For this review, take the finished solid that the model builds, in its own axes (mm). A direction names the side the tool comes from. Coordinates: 2 decimals unless noted, no trailing zeros. Loops run counter-clockwise (first coordinate to the right, second up) from the corner with the lowest first, then second, coordinate; pieces in that order, holes last. Notation, with made-up numbers: M 29,23.5 L 45,23.5 A17 cw 45,38.5 Z; hole C 32.25,49.25 d8. An arc over 180 degrees is marked long. Use one line per item in the form item = value.
```python
from build123d import *

# Parameters (mm, degrees)
FILLET1_R           = 11
FILLET2_R           = 1
BOSS_EXTRUDE1_DEPTH = 10.425
CHAMFER1_SIZE       = 0.35


with BuildPart() as part:
    # Sketch1 → Revolve1 (revolve)
    with BuildSketch(Plane.XY, mode=Mode.PRIVATE) as revolve1_sk:
        with BuildLine():
            Line((0, 0), (8.5, 0))
            Line((8.5, 0), (8.5, 1))
            Line((8.5, 1), (6, 8))
            Line((6, 8), (8, 23))
            Line((8, 23), (7.5, 24))
            Line((7.5, 24), (6.5, 24))
            add(Edge.make_bspline(
                [(6.5, 24), (3.269230769, 23.5), (0, 23.5)],
                knots=[0, 0, 0, 1, 1, 1], degree=2))
            Line((0, 23.5), (0, 0))
        make_face()
    revolve(revolve1_sk.sketch.rotate(Axis((0, 23.5, 0), (0, -1, 0)), 180), axis=Axis((0, 23.5, 0), (0, -1, 0)))

    # Fillet1
    fillet1_edges = [part.edges().sort_by_distance(p)[0] for p in [
        (6, 8, 0),
    ]]
    fillet(fillet1_edges, radius=FILLET1_R)

    # Fillet2
    fillet2_edges = [part.edges().sort_by_distance(p)[0] for p in [
        (6.5, 24, 0),
        (7.5, 24, 0),
        (8, 23, 0),
        (8.5, 1, 0),
    ]]
    fillet(fillet2_edges, radius=FILLET2_R)

    # Sketch3 → Cut-Revolve1 (revolve, cut)
    with BuildSketch(Plane.XY, mode=Mode.PRIVATE) as cut_revolve1_sk:
        Polygon((0, 0), (3.875, 0), (3.875, 6.5), (3.05, 7.325), (3.05, 17.75), (0, 17.75), align=None)
    revolve(cut_revolve1_sk.sketch.rotate(Axis((0, 17.75, 0), (0, -1, 0)), 180), axis=Axis((0, 17.75, 0), (0, -1, 0)), mode=Mode.SUBTRACT)

    # Sketch4 → Boss-Extrude1 (add)
    with BuildSketch(Plane.XZ.offset(-17.75)):
        with BuildLine():
            Line((-2.655654345, 1.5), (2.655654345, 1.5))
            ThreePointArc((2.655654345, 1.5), (0, 3.05), (-2.655654345, 1.5))
        make_face()
        with BuildLine():
            ThreePointArc((-0.099986562, -3.048360656), (0, -3.05), (0.099986562, -3.048360656))
            ThreePointArc((0.099986562, -3.048360656), (0, -2.95), (-0.099986562, -3.048360656))
        make_face()
    extrude(amount=BOSS_EXTRUDE1_DEPTH)

    # Chamfer1
    # the kernel refuses this chamfer: 0.35 mm, written as the material it takes off along each edge
    with BuildSketch(Plane(origin=(-3.555743391, 7.325, 1.5), x_dir=(0, -0.02749587661058614, 0.9996219169112968), z_dir=(1, 0, 0))) as chamfer1_piece_1_section:
        Polygon((CHAMFER1_SIZE * 0.999621916911, -CHAMFER1_SIZE * 0.0274958766106), (-CHAMFER1_SIZE * 0.0274958766106, -CHAMFER1_SIZE * 0.999621916911), (0, 0), align=None)
    chamfer1_piece_1 = extrude(amount=7.111486782, mode=Mode.PRIVATE)
    chamfer1_piece_1 = chamfer1_piece_1 & Plane(origin=(0, 7.499624527, 0), x_dir=(-1, 0, 0), z_dir=(0, 1, 0)) * Cylinder(3.05, 16, mode=Mode.PRIVATE)
    add(chamfer1_piece_1, mode=Mode.SUBTRACT)


solid = part.part
```
1. Consider section A-A on y = 13.5. Write out the cut boundary in (x, z), plus the area to 3 significant figures.
Computed values:
outline = C 0,0 d13.47; hole M -2.66,1.5 A3.05 ccw -0.1,-3.05 A0.1 cw 0.1,-3.05 A3.05 ccw 2.66,1.5 Z
area = 119 mm2
2. For pin 1 Ø4 at (x, y) = (-4.5, 19) entering from -Z; pin 2 Ø8 at (x, y) = (0, 20.5) entering from -Z; pin 3 Ø5 at (y, z) = (16, 4.5) entering from +X, all flat-tipped, find the tip position at first contact; note any pin that passes through.
Computed values:
pin_1 = -7.09
pin_2 = -7.97
pin_3 = 6.85
3. Draft analysis for pull direction X (two halves, no side actions). For faces 1 (the face through (-6.65, 5.28, -2.09)), 2 (the face through (0, 13, 1.5)), 3 (the face through (4, 0, 2)), state which applies: +X half, -X half, draft (parallel to the pull), parting line (faces both ways), or undercut.
Computed values:
face_1 = parting line
face_2 = undercut
face_3 = draft
4. Tool access review of faces 4 (the face through (-6.666, 15.414, -2.099)), 5 (the face through (1.107, 0.419, -8.428)), 6 (the face through (0, 7.325, 2)): name each direction out of +Z, -Z, +X, -X, +Y, -Y from which nothing blocks a thin tool from reaching the whole face with its end or side.
Computed values:
face_4 = none
face_5 = +Y, -Y
face_6 = -Y
5. Consider section B-B on y = 20.75. Write out the cut boundary in (x, z), plus the area to 3 significant figures.
Computed values:
outline = C 0,0 d15.4
area = 186 mm2
6. Wall thickness on line 1 along Z through (x, y) = (0, 5.25) (3 decimals); line 2 along X through (y, z) = (14.5, 1.25); line 3 along Y through (x, z) = (-0.5, 0.5): over which ranges is each line inside the solid? List them lowest first. Write a range as from..to.
Computed values:
line_1 = -6.982..-3.875, 3.875..6.982
line_2 = -6.75..-2.78, 2.78..6.75
line_3 = 17.75..23.51
